CAD build for the part. Positions are in the model's coordinates, mm. A direction names the side the tool comes from. Round coordinates to 2 decimals unless told otherwise and drop trailing zeros. Write each loop counter-clockwise with the first axis right and the second up, starting at its lowest first coordinate (ties: lowest second). Pieces come first, ordered by that corner, then holes. Notation, with made-up numbers: (-30, 39.5) - (-6, 39.5) arc R8 ccw to (-6, 54.5) - close; hole circle Ø9 at (12.5, 6.25). An arc over 180 degrees is marked (long way). Put each result on its own line as item: value. Start each with the question number.
Item 1: Mould opens along Y. For faces 1 (the flat face through (-20, 0, 2)), 2 (the cylindrical face through (16.995, 17.56, 53.535)), 3 (the flat face through (-13.838, 13.709, 27.678)) say: released by +Y, released by -Y, zero draft, split by the parting line, or undercut.
Item 2: Cut at B-B (z = 31). Give the cut face in (x, y).
Item 3: Cut at A-A (y = 0). Give the cut face in (x, z).
Item 4: Cut at D-D (x = 16). Count the separate pieces of the cut face and the enclosed holes in it, and give its area (3 significant figures).
Item 5: Pin check, flat tips, straight feed: pin 1 Ø8 at (y, z) = (2.5, 30.5) entering from -X; pin 2 Ø2 at (x, z) = (-14.5, 27) entering from +Y; pin 3 Ø13 at (x, z) = (0, 15.5) entering from +Y. Stop position of each tip, or through.
Item 6: 3-axis set-ups, long thin cutter, end or side, ignore diameter. For faces 4 (the flat face through (19, 0, 28)), 5 (the cylindrical face through (18.844, -8.494, 28.322)), 6 (the flat face through (-19.4, 0.1, 5)), 7 (the cylindrical face through (18.852, 8.474, 28.322)), 8 (the cylindrical face through (-8.494, -18.844, 28.322)): which of +Z, -Z, +X, -X, +Y, -Y reach the whole face in a straight line?
Item 7: Drill centre lines: line 1 (X direction, y = 1.5, z = 20); line 2 (Y direction, x = -16, z = 53.5); line 3 (X direction, y = -6, z = 53). Where is each one in solid material? Low to high. Write a range as from..to.
Autodesk Inventor part; units mm, degrees
ref_plane "YZ Plane" through (0, 0, 0) normal (1, 0, 0) x (0, 1, 0)
ref_plane "XZ Plane" through (0, 0, 0) normal (0, 1, 0) x (-1, 0, 0)
ref_plane "XY Plane" through (0, 0, 0) normal (0, 0, 1) x (1, 0, 0)
sketch "Sketch1" plane through (0, 0, 0) normal (0, 0, 1) x (1, 0, 0)
  line L0 (20, -20) -> (-20, -20)
  line L1 (-20, -20) -> (-20, 20)
  line L2 (-20, 20) -> (20, 20)
  line L3 (20, 20) -> (20, -20)
  line L4 (20, -20) -> (-20, 20) construction
  line L5 (-20, -20) -> (20, 20) construction
  point P0 (0, 0)
  dimension "d0" = 40
  dimension "d1" = 40
extrude "Extrusion1" add sketch "Sketch1" along normal blind 5
sketch "Sketch2" plane through (0, 0, 5) normal (0, 0, 1) x (1, 0, 0)
  line L0 (20, 20) -> (-20, 20)
  line L1 (-20, 20) -> (-20, -20)
  line L2 (8.547, -19) -> (-8.547, -19)
  line L3 (-19, -8.547) -> (-19, 8.547)
  line L4 (-8.547, 19) -> (8.547, 19)
  line L5 (19, 8.547) -> (19, -8.547)
  line L6 (19, -19) -> (-19, 19) construction
  line L7 (-19, -19) -> (19, 19) construction
  line L8 (19, 6.0309) -> (19, -12.9361)
  line L9 (-19, 8.547) -> (-8.547, 19)
  line L10 (8.547, 19) -> (19, 8.547)
  line L11 (19, -8.547) -> (8.547, -19)
  line L12 (-8.547, -19) -> (-19, -8.547)
  point P0 (0, 0)
  dimension "d16" = 38
  dimension "d17" = 38
  dimension "d18" = 10.453
  dimension "d19" = 10.453
  dimension "d20" = 10.453
  dimension "d21" = 10.453
  dimension "d22" = 10.453
  dimension "d23" = 10.453
  dimension "d24" = 10.453
  dimension "d25" = 10.453
extrude "Extrusion2" add sketch "Sketch2" along normal blind 46
sketch "Sketch3" plane through (0, 0, 51) normal (0, 0, 1) x (1, 0, 0)
  line L0 (20, 20) -> (-20, 20)
  line L1 (20, -20) -> (-20, -20)
  line L2 (-20, -20) -> (-20, 20)
  line L3 (-20, 20) -> (20, 20)
  line L4 (20, 20) -> (20, -20)
  line L5 (20, -20) -> (-20, 20) construction
  line L6 (-20, -20) -> (20, 20) construction
  point P0 (0, 0)
extrude "Extrusion3" add sketch "Sketch3" along normal blind 5
sketch "Sketch5" plane through (0, 0, 56) normal (0, 0, 1) x (1, 0, 0)
  line L0 (8, -18.5) -> (-8, -18.5)
  line L1 (-18.5, -8) -> (-18.5, 8)
  line L2 (-8, 18.5) -> (8, 18.5)
  line L3 (18.5, 8) -> (18.5, -8)
  line L4 (18.5, -18.5) -> (-18.5, 18.5) construction
  line L5 (-18.5, -18.5) -> (18.5, 18.5) construction
  line L6 (-18.5, 8) -> (-8, 18.5)
  line L7 (8, 18.5) -> (18.5, 8)
  line L8 (18.5, -8) -> (8, -18.5)
  line L9 (-18.5, -8) -> (-8, -18.5)
  point P0 (0, 0)
  dimension "d27" = 37
  dimension "d28" = 37
  dimension "d29" = 10.5
  dimension "d30" = 10.5
  dimension "d31" = 10.5
  dimension "d32" = 10.5
  dimension "d33" = 10.5
  dimension "d34" = 10.5
  dimension "d35" = 10.5
  dimension "d36" = 10.5
extrude "Extrusion5" cut sketch "Sketch5" against normal through all
fillet "Fillet2" radius 2 16 edges at (20, 20, 53.5) (20, 20, 2.5) (-20, 20, 53.5) (-20, 20, 2.5) (-20, -20, 53.5) (-20, -20, 2.5) (20, -20, 53.5) (20, -20, 2.5) (19, -8.547, 28) (8.547, -19, 28) (-8.547, -19, 28) (-19, -8.547, 28) (-19, 8.547, 28) (-8.547, 19, 28) (8.547, 19, 28) (19, 8.547, 28)
sketch "Sketch6" plane through (0, 0, 56) normal (0, 0, 1) x (1, 0, 0)
  line L0 (-16, -16) -> (16, -16) construction
  line L1 (16, -16) -> (16, 16) construction
  line L2 (16, 16) -> (-16, 16) construction
  line L3 (-16, 16) -> (-16, -16) construction
  line L4 (-16, -16) -> (16, 16) construction
  line L5 (16, -16) -> (-16, 16) construction
  circle A0 centre (16, 16) radius 1.85
  circle A1 centre (16, -16) radius 1.85
  circle A2 centre (-16, -16) radius 1.85
  circle A3 centre (-16, 16) radius 1.85
  point P0 (0, 0)
  dimension "d40" = 32
  dimension "d41" = 32
  dimension "d42" = 3.7
  dimension "d43" = 3.7
  dimension "d44" = 3.7
  dimension "d45" = 3.7
extrude "Extrusion6" cut sketch "Sketch6" against normal blind 56
equation "\"d19\" = d18"
equation "\"d20\" = d18"
equation "\"d21\" = d20"
equation "\"d22\" = d18"
equation "\"d23\" = d22"
equation "\"d24\" = d18"
equation "\"d25\" = d24"
equation "\"d30\" = d29"
equation "\"d31\" = d29"
equation "\"d32\" = d31"
equation "\"d33\" = d29"
equation "\"d34\" = d33"
equation "\"d35\" = d29"
equation "\"d36\" = d35"
properties part number "fan"
Output values:
1. face 1: zero draft
1. face 2: undercut
1. face 3: released by +Y
2. outline: (-19, -7.72) arc R2 ccw to (-18.41, -9.13) - (-9.13, -18.41) arc R2 ccw to (-7.72, -19) - (7.72, -19) arc R2 ccw to (9.13, -18.41) - (18.41, -9.13) arc R2 ccw to (19, -7.72) - (19, 7.72) arc R2 ccw to (18.41, 9.13) - (9.13, 18.41) arc R2 ccw to (7.72, 19) - (-7.72, 19) arc R2 ccw to (-9.13, 18.41) - (-18.41, 9.13) arc R2 ccw to (-19, 7.72) - close; hole (-18.5, -8) - (-8, -18.5) - (8, -18.5) - (18.5, -8) - (18.5, 8) - (8, 18.5) - (-8, 18.5) - (-18.5, 8) - close
3. outline: (-20, 0) - (-18.5, 0) - (-18.5, 56) - (-20, 56) - (-20, 51) - (-19, 51) - (-19, 5) - (-20, 5) - close; (18.5, 0) - (20, 0) - (20, 5) - (19, 5) - (19, 51) - (20, 51) - (20, 56) - (18.5, 56) - close
4. separate pieces: 6
4. enclosed holes: 0
4. area: 212 mm2
5. pin 1: x = -19
5. pin 2: y = 14.05
5. pin 3: y = 19
6. face 4: +X, +Y, -Y
6. face 5: +X, -Y
6. face 6: none
6. face 7: +X, +Y
6. face 8: -X, -Y
7. line 1: -19..-18.5, 18.5..19
7. line 2: -20..-17.85, -14.15..-10.5, 10.5..14.15, 17.85..20
7. line 3: -20..-18.5, 18.5..20
